```python
from build123d import *

# Parameters (mm, degrees)
SKETCH1_W           = 6.25
SKETCH1_H           = 2.5
SKETCH1_W_2         = 8.8
BOSS_EXTRUDE1_DEPTH = 45
SKETCH9_W           = 26
SKETCH9_H           = 7.5
BOSS_EXTRUDE3_DEPTH = 3
SKETCH10_W          = 11.15
SKETCH10_H          = 48
CUT_EXTRUDE3_DEPTH  = 1


with BuildPart() as part:
    # Sketch1 → Boss-Extrude1 (new body)
    with BuildSketch(Plane.XY):
        Polygon((-3.202898551, 2.789855072), (-3.202898551, 0.289855072), (3.047101449, 0.289855072), (9.797101449, 0.289855072), (9.797101449, 2.789855072), align=None)
        with Locations((-0.077898551, -0.960144928)):
            Rectangle(SKETCH1_W, SKETCH1_H)
        with Locations((1.197101449, -3.460144928)):
            Rectangle(SKETCH1_W_2, SKETCH1_H)
    boss_extrude1 = extrude(amount=BOSS_EXTRUDE1_DEPTH)

    # Mirror1: Boss-Extrude1 across plane
    add(boss_extrude1.mirror(Plane(origin=(-3.202898551, 0, 45), x_dir=(0, 0, 1), z_dir=(-1, 0, 0))))

    # Cut-Extrude2 cone 1 section (through the dimple's axis) → Cut-Extrude2 (revolve, cut)
    with BuildSketch(Plane(origin=(-3.202898551, -4.710144928, 32.5), x_dir=(0, 0, -1), z_dir=(1, 0, 0))):
        Polygon((0, 0), (1.5, 0), (0, 1.5), align=None)
    revolve(axis=Axis((-3.202898551, -4.710144928, 32.5), (0, 1, 0)), mode=Mode.SUBTRACT)

    # Cut-Extrude2 cone 2 section (through the dimple's axis) → Cut-Extrude2 cone 2 (revolve, cut)
    with BuildSketch(Plane(origin=(-3.202898551, -4.710144928, 12.5), x_dir=(0, 0, -1), z_dir=(1, 0, 0))):
        Polygon((0, 0), (1.5, 0), (0, 1.5), align=None)
    revolve(axis=Axis((-3.202898551, -4.710144928, 12.5), (0, 1, 0)), mode=Mode.SUBTRACT)

    # Sketch9 → Boss-Extrude3 (add)
    with BuildSketch(Plane(origin=(0, 0, 0), x_dir=(-1, 0, 0), z_dir=(0, 0, -1))):
        with Locations((3.202898551, -0.960144928)):
            Rectangle(SKETCH9_W, SKETCH9_H)
    extrude(amount=BOSS_EXTRUDE3_DEPTH)

    # Sketch10 → Cut-Extrude3 (cut)
    with BuildSketch(Plane(origin=(0, 2.789855072, 0), x_dir=(1, 0, 0), z_dir=(0, 1, 0))):
        with Locations((-8.777898551, -21)):
            Rectangle(SKETCH10_W, SKETCH10_H)
        with Locations((2.372101449, -21)):
            Rectangle(SKETCH10_W, SKETCH10_H)
    extrude(amount=-CUT_EXTRUDE3_DEPTH, mode=Mode.SUBTRACT)


solid = part.part
```
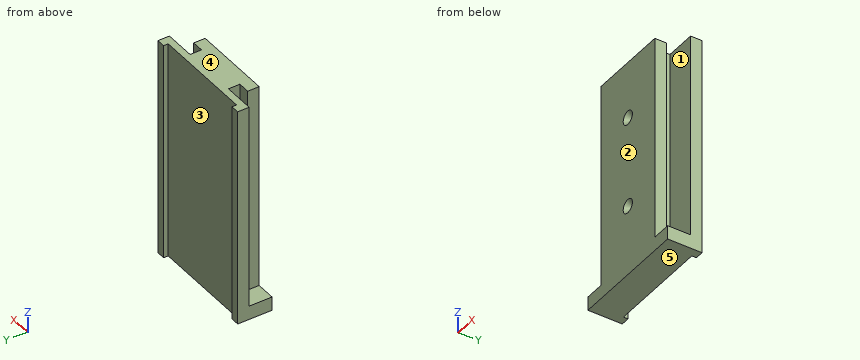
Source: CAD feature listing. Evaluate the final solid. Frame: model axes, mm. Face numbers are marked on the shaded views. A direction names the side the tool comes from. Round coordinates to 2 decimals unless told otherwise and drop trailing zeros. Write each loop counter-clockwise with the first axis right and the second up, starting at its lowest first coordinate (ties: lowest second). Pieces come first, ordered by that corner, then holes. Notation, with made-up numbers: M -12.75,-31.5 L 44.25,-31.5 A16 cw 44.25,-25.5 Z; hole C 37.25,-37 d1. An arc over 180 degrees is marked long. Answer as a JSON object with one key per item and string values. Group by question number.
(1) Reachability of the marked faces 1 and 2 from +Z, -Z, +X, -X, +Y, -Y: full face, straight path, thin tool, end or side. Return the list, or none.
(2) Ray query, line 1 (Y direction, x = 4.25, z = 9); line 2 (Y direction, x = -4, z = 27); line 3 (X direction, y = -0.25, z = 3.5). Return the intervals inside material, ascending. Write a range as [from, to].
(3) First-contact query: pin 1 (2 mm diameter, centred on x = -10.5, z = 23.5, fed in from +Y); pin 2 (2.5 mm diameter, centred on x = 7.5, y = -2, fed in from +Z); pin 3 (0.8 mm diameter, centred on y = -1.5, z = 16, fed in from -X). Flat tips, straight axial feed; report the tip coordinate or a pass-through.
(4) Section query C-C on x = -7. Output: boundary loops of the cut face in (y, z).
(5) Section query B-B on x = -10. Output: boundary loops of the cut face in (y, z), then the cut area to 4 significant figures.
(6) Mould query, pull axis Z, two halves, no side actions, for the marked faces 3, 4 and 5. Classes: +Z half, -Z half, draft (parallel to the pull), parting line (faces both ways), or undercut.
(7) Section query A-A on y = -1. Output: boundary loops of the cut face in (x, z), then the cut area to 4 significant figures.
Computed values:
{
 "1": {"face 1": "+Z, +X", "face 2": "+Z, -Z, +X, -X, -Y"},
 "2": {"line 1": "[-4.71, -2.21], [0.29, 1.79]", "line 2": "[-4.71, 1.79]", "line 3": "[-9.45, 3.05]"},
 "3": {"pin 1": "y = 1.79", "pin 2": "z = 0", "pin 3": "x = -9.45"},
 "4": {"outline": "M -4.71,-3 L 1.79,-3 L 1.79,45 L -4.71,45 Z"},
 "5": {"outline": "M -4.71,-3 L 1.79,-3 L 1.79,45 L 0.29,45 L 0.29,0 L -2.21,0 L -2.21,45 L -4.71,45 Z", "area": "199.5 mm^2"},
 "6": {"face 3": "draft", "face 4": "+Z half", "face 5": "-Z half"},
 "7": {"outline": "M -16.2,-3 L 9.8,-3 L 9.8,0 L 3.05,0 L 3.05,45 L -9.45,45 L -9.45,0 L -16.2,0 Z", "area": "640.5 mm^2"}
}
